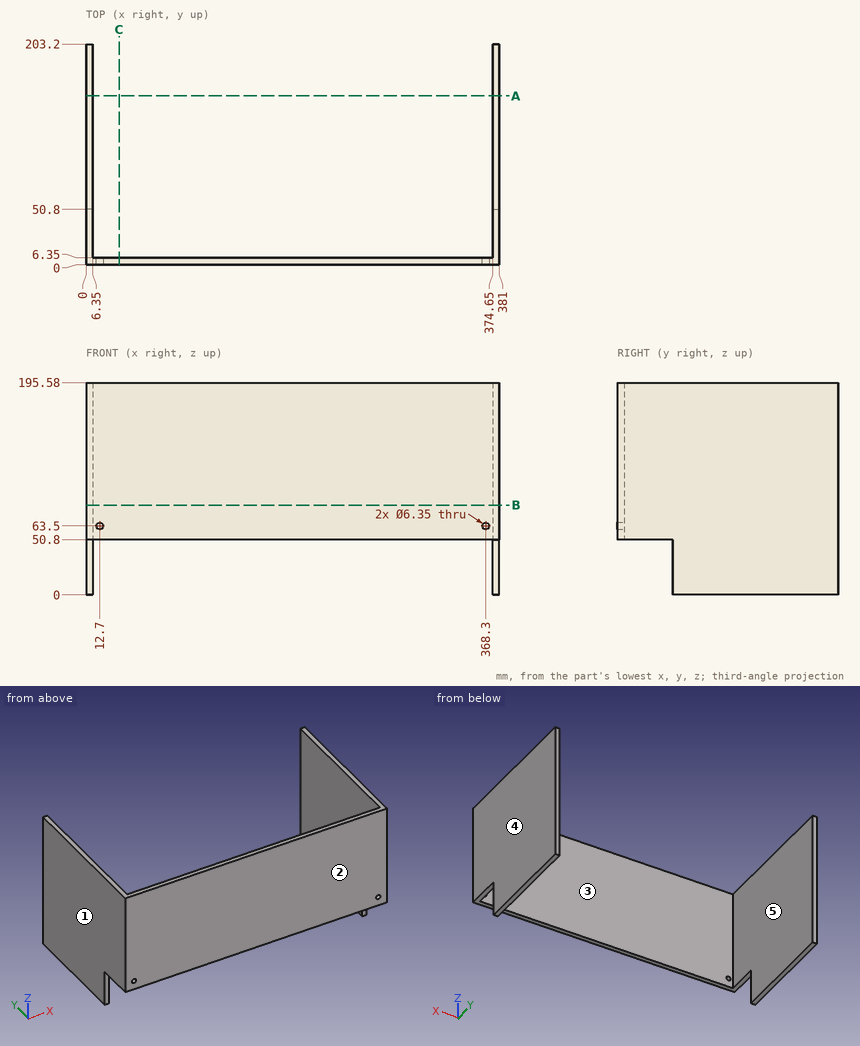
Geometry: see drawing. Coordinates: mm, zero at the bounding-box minimum. A direction names the side the tool comes from. Give positions to 0.01 mm unless a question says otherwise; leave off trailing zeros. Loops run counter-clockwise (first coordinate to the right, second up) from the corner with the lowest first, then second, coordinate; pieces in that order, holes last. Notation, with made-up numbers: (28, -32.75) -> (80, -32.75) arc R20 cw to (80, -14.75) -> close; hole circle Ø8 at (60.25, 20.25). An arc over 180 degrees is marked (long way). Use one line per item in the form item = value.
Item 1: Access query for the marked faces 4 and 5. Directions: +Z, -Z, +X, -X, +Y, -Y. A direction counts if a zero-diameter tool reaches every point of the face in a straight line with its end or side. Return the directions, or none.
A:
face_4 = +Z, -Z, +X, +Y, -Y
face_5 = +Z, -Z, +Y
Item 2: Section query B-B on z = 82.5. Output: boundary loops of the cut face in (x, y).
A:
outline = (0, 0) -> (381, 0) -> (381, 203.2) -> (374.65, 203.2) -> (374.65, 6.35) -> (6.35, 6.35) -> (6.35, 203.2) -> (0, 203.2) -> close
Item 3: Section query A-A on y = 155.5. Output: boundary loops of the cut face in (x, z), and give its area (3 significant figures).
A:
outline = (0, 0) -> (6.35, 0) -> (6.35, 195.58) -> (0, 195.58) -> close; (374.65, 0) -> (381, 0) -> (381, 195.58) -> (374.65, 195.58) -> close
area = 2,480 mm^2
Item 4: Pin query (flat end, axial travel): P1, Ø7, axis at x = 3, z = 14, coming from the -Y side; P2, Ø3, axis at x = 107, z = 112.5, coming from the +Y side; P3, Ø5.5, axis at x = 12.7, z = 63.5, coming from the -Y side. Return the tip coordinate at first contact, or that it passes through.
A:
P1 = 50.8
P2 = 6.35
P3 = through
Item 5: Section query C-C on x = 30.5. Output: boundary loops of the cut face in (y, z).
A:
outline = (0, 50.8) -> (6.35, 50.8) -> (6.35, 195.58) -> (0, 195.58) -> close
Item 6: Draft query along X for the marked faces 1, 2 and 3. Return one class per face: pulls with the +X half, pulls with the -X half, needs draft (parallel to the pull), parting line crosses it, or undercut.
A:
face_1 = pulls with the -X half
face_2 = needs draft
face_3 = undercut
Item 7: Line query: probe 1 along X at (y, z) = (4.5, 63.5) (3 decimals); probe 2 along X at (y, z) = (77.5, 171); probe 3 along Z at (x, y) = (368.3, 3.75) (3 decimals). Output: solid intervals per line, ascending.
A:
probe_1 = 0 to 9.525, 15.875 to 365.125, 371.475 to 381
probe_2 = 0 to 6.35, 374.65 to 381
probe_3 = 50.8 to 60.325, 66.675 to 195.58
